Autodesk Inventor part; units mm, degrees
ref_plane "YZ Plane" through (0, 0, 0) normal (1, 0, 0) x (0, 1, 0)
ref_plane "XZ Plane" through (0, 0, 0) normal (0, 1, 0) x (-1, 0, 0)
ref_plane "XY Plane" through (0, 0, 0) normal (0, 0, 1) x (1, 0, 0)
sketch "スケッチ1" plane through (0, 0, 0) normal (0, 0, 1) x (1, 0, 0)
  circle A0 centre (110.4743, -16.4118) radius 30.1 construction
  circle A1 centre (150.4743, 0.5882) radius 1.5
  circle A2 centre (127.6431, 30.2622) radius 1.5
  circle A3 centre (80.4743, 23.124) radius 1.5
  circle A4 centre (70.4743, -10.4118) radius 1.5
  circle A5 centre (110.4743, -16.4118) radius 7.025
  arc A6 (79.801, 27.5733) -> (76.162, 24.4099) centre (80.4743, 23.124) ccw
  arc A7 (131.2097, 33.0062) -> (126.9698, 34.7115) centre (127.6431, 30.2622) ccw
  arc A8 (154.401, -1.6098) -> (154.0408, 3.3323) centre (150.4743, 0.5882) ccw
  arc A9 (66.162, -9.1259) -> (66.7172, -12.8885) centre (70.4743, -10.4118) ccw
  arc A10 (117.3199, -46.749) -> (137.6119, -31.6026) centre (110.4743, -16.4118) ccw
  line L0 (154.401, -1.6098) -> (137.6119, -31.6026)
  line L1 (66.162, -9.1259) -> (76.162, 24.4099)
  line L2 (79.801, 27.5733) -> (126.9698, 34.7115)
  line L3 (131.2097, 33.0062) -> (154.0408, 3.3323)
  line L4 (96.5433, 16.3458) -> (118.2214, -10.0492) construction
  line L5 (117.0311, -23.9953) -> (91.1935, -46.3348) construction
  circle A11 centre (100.1953, 16.6261) radius 3 construction
  circle A12 centre (144.4932, -10.0968) radius 3 construction
  circle A13 centre (100.1953, 16.6261) radius 4.5 construction
  circle A14 centre (144.4932, -10.0968) radius 4.5 construction
  arc A15 (90.988, -49.7066) -> (95.7356, -51.6195) centre (94.7451, -47.2298) ccw
  circle A16 centre (94.7451, -47.2298) radius 3 construction
  line L6 (95.7356, -51.6195) -> (117.3199, -46.749)
  line L7 (66.7172, -12.8885) -> (90.988, -49.7066)
  circle A17 centre (100.1953, 16.6261) radius 1.25
  circle A18 centre (144.4932, -10.0968) radius 1.25
  circle A19 centre (94.7451, -47.2298) radius 1.25
  point P0 (0, 0)
  point P1 (0, 0)
  point P2 (0, 0)
  dimension "d0" = 14.05
  dimension "d1" = 9
  dimension "d2" = 9
  dimension "d3" = 9
  dimension "d4" = 9
  dimension "d5" = 1
  dimension "d6" = 6
  dimension "d7" = 6
  dimension "d8" = 9
  dimension "d9" = 9
  dimension "d10" = 9
  dimension "d11" = 6
  dimension "d12" = 2.5
  dimension "d13" = 2.5
  dimension "d14" = 2.5
sketch "スケッチ2" plane through (0, 0, 0) normal (0, 0, 1) x (1, 0, 0)
  circle A0 centre (100.1953, 16.6261) radius 1.25
  circle A1 centre (144.4932, -10.0968) radius 1.25
  circle A2 centre (94.7451, -47.2298) radius 1.25
  line L0 (95.7356, -51.6195) -> (117.3199, -46.749)
  arc A3 (117.3199, -46.749) -> (137.6119, -31.6026) centre (110.4743, -16.4118) ccw
  line L1 (154.401, -1.6098) -> (137.6119, -31.6026)
  arc A4 (90.988, -49.7066) -> (95.7356, -51.6195) centre (94.7451, -47.2298) ccw
  arc A5 (102.5197, 20.4792) -> (95.7116, 17.0088) centre (100.1953, 16.6261) ccw
  arc A6 (148.4198, -12.2949) -> (146.8176, -6.2437) centre (144.4932, -10.0968) ccw
  line L2 (148.4198, -12.2949) -> (137.6119, -31.6026)
  arc A7 (90.2614, -46.8472) -> (90.988, -49.7066) centre (94.7451, -47.2298) ccw
  line L3 (90.2614, -46.8472) -> (95.7116, 17.0088)
  line L4 (102.5197, 20.4792) -> (146.8176, -6.2437)
  circle A8 centre (110.4743, -16.4118) radius 7.025
  point P0 (0, 0)
  dimension "d15" = 9
  dimension "d16" = 9
extrude "押し出し1" add sketch "スケッチ2" along normal blind 3
sketch "スケッチ3" plane through (0, 0, 3) normal (0, 0, 1) x (1, 0, 0)
  circle A0 centre (110.4743, -16.4118) radius 7.025
  circle A1 centre (94.7451, -47.2298) radius 1.25
  circle A2 centre (144.4932, -10.0968) radius 1.25
  circle A3 centre (100.1953, 16.6261) radius 1.25
  line L0 (95.7356, -51.6195) -> (117.3199, -46.749)
  arc A4 (117.3199, -46.749) -> (137.6119, -31.6026) centre (110.4743, -16.4118) ccw
  line L1 (137.6119, -31.6026) -> (148.4198, -12.2949)
  arc A5 (148.4198, -12.2949) -> (146.8176, -6.2437) centre (144.4932, -10.0968) ccw
  line L2 (146.8176, -6.2437) -> (102.5197, 20.4792)
  arc A6 (102.5197, 20.4792) -> (95.7116, 17.0088) centre (100.1953, 16.6261) ccw
  line L3 (95.7116, 17.0088) -> (90.2614, -46.8472)
  arc A7 (90.2614, -46.8472) -> (95.7356, -51.6195) centre (94.7451, -47.2298) ccw
  line L4 (100.9701, 17.9105) -> (145.268, -8.8124)
  arc A8 (145.8021, -10.8295) -> (145.268, -8.8124) centre (144.4932, -10.0968) ccw
  line L5 (145.8021, -10.8295) -> (134.9942, -30.1373)
  arc A9 (116.6595, -43.8226) -> (134.9942, -30.1373) centre (110.4743, -16.4118) ccw
  line L6 (116.6595, -43.8226) -> (95.0753, -48.6931)
  arc A10 (93.2506, -47.1023) -> (95.0753, -48.6931) centre (94.7451, -47.2298) ccw
  line L7 (93.2506, -47.1023) -> (98.7007, 16.7536)
  arc A11 (100.9701, 17.9105) -> (98.7007, 16.7536) centre (100.1953, 16.6261) ccw
  circle A12 centre (110.4743, -16.4118) radius 10.025
  arc A13 (98.3399, 12.5264) -> (104.6029, 15.719) centre (100.1953, 16.6261) ccw
  circle A14 centre (144.4932, -10.0968) radius 1.25
  arc A15 (141.6352, -6.6209) -> (143.7297, -14.5316) centre (144.4932, -10.0968) ccw
  arc A16 (99.2139, -47.7592) -> (93.6114, -42.875) centre (94.7451, -47.2298) ccw
  circle A17 centre (94.7451, -47.2298) radius 1.5
  circle A18 centre (144.4932, -10.0968) radius 1.5
  circle A19 centre (100.1953, 16.6261) radius 1.5
  line L8 (110.4743, -16.4118) -> (144.4932, -10.0968) construction
  arc A20 (110.2006, -14.937) -> (110.7481, -17.8866) centre (110.4743, -16.4118) ccw
  arc A21 (144.7669, -11.5716) -> (144.2194, -8.622) centre (144.4932, -10.0968) ccw
  line L9 (100.1953, 16.6261) -> (110.4743, -16.4118) construction
  arc A22 (101.6276, 17.0717) -> (98.763, 16.1804) centre (100.1953, 16.6261) ccw
  arc A23 (109.0421, -16.8574) -> (111.9066, -15.9662) centre (110.4743, -16.4118) ccw
  line L10 (110.4743, -16.4118) -> (94.7451, -47.2298) construction
  arc A24 (111.8104, -17.0937) -> (109.1383, -15.7299) centre (110.4743, -16.4118) ccw
  arc A25 (93.4091, -46.5479) -> (96.0812, -47.9118) centre (94.7451, -47.2298) ccw
  line L11 (110.7481, -17.8866) -> (117.4958, -16.634)
  line L12 (120.4938, -16.0775) -> (140.5956, -12.346)
  line L13 (140.048, -9.3964) -> (119.9462, -13.1279)
  line L14 (116.9483, -13.6844) -> (110.2006, -14.937)
  line L15 (111.9066, -15.9662) -> (109.8677, -9.413)
  line L16 (108.9619, -6.5015) -> (102.888, 13.0206)
  line L17 (100.0234, 12.1294) -> (106.0973, -7.3928)
  line L18 (107.0032, -10.3043) -> (109.0421, -16.8574)
  line L19 (109.1383, -15.7299) -> (108.8606, -16.2741)
  line L20 (104.6322, -24.5586) -> (95.3378, -42.769)
  line L21 (98.0099, -44.1329) -> (107.3043, -25.9224)
  line L22 (108.6904, -23.2065) -> (111.8104, -17.0937)
  point P0 (0, 0)
  point P1 (127.4837, -13.2543)
  point P2 (105.3348, 0.1071)
  point P3 (102.6097, -31.8208)
  dimension "d20" = 3
  dimension "d21" = 3
  dimension "d22" = 3
  dimension "d23" = 3
  dimension "d24" = 3
  dimension "d25" = 3
  dimension "d26" = 3
  dimension "d27" = 3
  dimension "d28" = 3
  dimension "d29" = 3
  dimension "d30" = 3
extrude "押し出し2" cut sketch "スケッチ3" against normal blind 2.5 contours L4 A15 L13 A12 L16 A13 | A13 L17 A12 L20 A16 L7 | A15 L5 A9 L6 A16 L21 A12 L12
extrude "押し出し3" cut sketch "スケッチ3" against normal blind 3 contours A19 A11 | A8 A18 | A17 A10
fillet "フィレット1" radius 1 18 edges at (104.6029, 15.719, 1.75) (102.888, 13.0206, 1.75) (100.0234, 12.1294, 1.75) (98.3399, 12.5264, 1.75) (106.0973, -7.3928, 1.75) (108.9619, -6.5015, 1.75) (119.9462, -13.1279, 1.75) (120.4938, -16.0775, 1.75) (107.3043, -25.9224, 1.75) (104.6322, -24.5586, 1.75) (95.3378, -42.769, 1.75) (93.6114, -42.875, 1.75) (98.0099, -44.1329, 1.75) (99.2139, -47.7592, 1.75) (143.7297, -14.5316, 1.75) (140.5956, -12.346, 1.75) (140.048, -9.3964, 1.75) (141.6352, -6.6209, 1.75)
properties part number "前足ギアトレイン抑え" material "ポリカーボネート、クリア"
The model under review builds one solid part; all positions refer to its coordinate system, in mm. A direction names the side the tool comes from. Give positions to 0.01 mm unless a question says otherwise; leave off trailing zeros. Write each loop counter-clockwise with the first axis right and the second up, starting at its lowest first coordinate (ties: lowest second). Pieces come first, ordered by that corner, then holes. Notation, with made-up numbers: (-1.75, 4) - (55.25, 4) arc R28 cw to (55.25, 40) - close; hole circle Ø6 at (-10.75, 45). An arc over 180 degrees is marked (long way). Answer in a Markdown table with one row per item. Add a question column.
1. We need section C-C on y = -28. Write out the cut boundary in (x, z), then the cut area to 3 significant figures.
2. We need section A-A on x = 115. Write out the cut boundary in (y, z).
3. We need section D-D on z = 1.8. State how many separate pieces and enclosed holes the cut face has, then the cut area to 3 significant figures.
4. We need section B-B on x = 128.5. Write out the cut boundary in (y, z), then the cut area to 3 significant figures.
5. Draft analysis for pull direction X (two halves, no side actions). For faces 1 (the cylindrical face through (141.696, -13.622, 1.768)), 2 (the cylindrical face through (98.095, 20.606, 1.479)), 3 (the flat face through (117, -21, 3)), 4 (the cylindrical face through (129.223, -41.225, 1.479)), state which applies: +X half, -X half, draft (parallel to the pull), parting line (faces both ways), or undercut.
6. Insertion check: P1, Ø6, axis at x = 105, y = -38.5, coming from the +Z side; P2, Ø2.5, axis at x = 100.2, y = 16.63, coming from the -Z side; P3, Ø5, axis at x = 115.5, y = -31.5, coming from the -Z side; P4, Ø1.5, axis at x = 98, z = 2.5, coming from the -Y side. Each pin has a flat end and moves straight along its axis. Give the tip position at first contact, or say it passes through.
7. Tool access review of faces 5 (the flat face through (92.95, -15.37, 1.48)), 6 (the cylindrical face through (115.726, -7.873, 1.768)), 7 (the cylindrical face through (99.53, 17.97, 1.52)): name each direction out of +Z, -Z, +X, -X, +Y, -Y from which nothing blocks a thin tool from reaching the whole face with its end or side.
8. Wall thickness on line 1 along X through (y, z) = (-9, 1.3); line 2 along X through (y, z) = (-4, 1.2); line 3 along Y through (x, z) = (116, 1.2): over which ranges is each line inside the solid? List them lowest first. Write a range as [from, to].
Ans:
| question | item | result |
|---|---|---|
| 1 | outline | (91.87, 0) - (139.63, 0) - (139.63, 3) - (136.19, 3) - (136.19, 0.5) - (106.24, 0.5) - (106.24, 3) - (102.88, 3) - (102.88, 0.5) - (94.88, 0.5) - (94.88, 3) - (91.87, 3) - close |
| 1 | area | 48.4 mm^2 |
| 2 | outline | (-47.27, 0) - (-21.78, 0) - (-21.78, 3) - (-25.36, 3) - (-25.36, 0.5) - (-44.2, 0.5) - (-44.2, 3) - (-47.27, 3) - close; (-11.04, 0) - (12.95, 0) - (12.95, 3) - (9.45, 3) - (9.45, 0.5) - (-7.47, 0.5) - (-7.47, 3) - (-11.04, 3) - close |
| 3 | separate pieces | 1 |
| 3 | enclosed holes | 7 |
| 3 | area | 1,010 mm^2 |
| 4 | outline | (-41.76, 0) - (4.81, 0) - (4.81, 3) - (1.3, 3) - (1.3, 0.5) - (-11.54, 0.5) - (-11.54, 3) - (-14.59, 3) - (-14.59, 0.5) - (-37.97, 0.5) - (-37.97, 3) - (-41.76, 3) - close |
| 4 | area | 49.1 mm^2 |
| 5 | face 1 | undercut |
| 5 | face 2 | parting line |
| 5 | face 3 | draft |
| 5 | face 4 | +X half |
| 6 | P1 | stops at z = 0.5 |
| 6 | P2 | passes through |
| 6 | P3 | stops at z = 0 |
| 6 | P4 | stops at y = -51.28 |
| 7 | face 5 | +Z, -Z, -X, +Y |
| 7 | face 6 | +Z |
| 7 | face 7 | +Z, -Z |
| 8 | line 1 | x = [93.49, 96.5], [103.72, 117.22], [140.1, 143.47], [145.52, 148.86] |
| 8 | line 2 | x = [93.92, 96.93], [105.04, 108.18], [137.29, 143.1] |
| 8 | line 3 | y = [-47.05, -43.97], [-24.78, -20.75], [-12.07, -8.05], [8.84, 12.35] |
